Work out the finished part from the listing and answer in its coordinate system (mm). Face numbers are marked on the shaded views. A direction names the side the tool comes from. Round coordinates to 2 decimals unless told otherwise and drop trailing zeros. Loops run counter-clockwise (first coordinate to the right, second up) from the corner with the lowest first, then second, coordinate; pieces in that order, holes last. Notation, with made-up numbers: (-11.5, -35) -> (45.5, -35) arc R27 ccw to (45.5, -2) -> close; hole circle Ø10 at (11, 32.25). An arc over 180 degrees is marked (long way). Use one line per item in the form item = value.
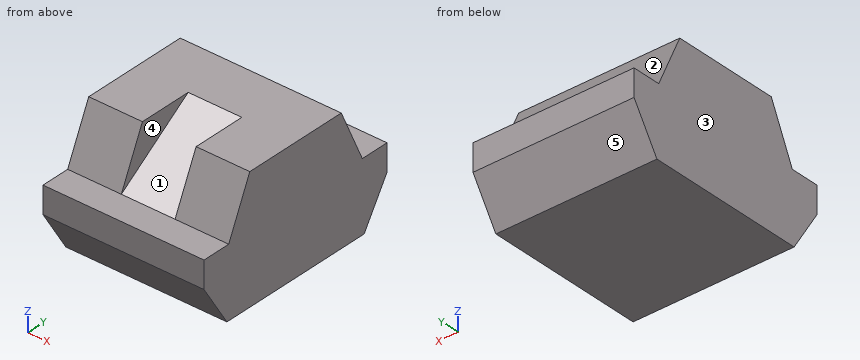
```python
from build123d import *

# Parameters (mm, degrees)
F1_DEPTH      = 76.2
F4_DEPTH      = 12.7
F4_DEPTH_BACK = 12.7


with BuildPart() as f1:
    # F0 (on Right) → F1 (new body)
    with BuildSketch(Plane.YZ):
        Polygon((-38.1, 0), (0, 0), (0, 58.3063843763), (-25.4, 58.3063843763), (-37.1005810608, 32.9063843763), (-50.8005463281, 32.9057950318), (-50.8, 20.2057950318), align=None)
        Polygon((0, 58.3063843763), (0, 0), (38.1, 0), (50.8, 20.2057950318), (50.8005463281, 32.9057950318), (37.1005810608, 32.9063843763), (25.4, 58.3063843763), align=None)
    extrude(amount=F1_DEPTH)

    # F3 (on mid) → F4 (cut, two sides)
    with BuildSketch(Plane.YZ.offset(38.1)) as f4_sk:
        Polygon((0, 58.3063843763), (-25.4, 58.3063843763), (-37.1005810608, 32.9063843763), align=None)
    extrude(amount=-F4_DEPTH, mode=Mode.SUBTRACT)
    extrude(f4_sk.sketch, amount=F4_DEPTH_BACK, mode=Mode.SUBTRACT)


solid = f1.part
```
(1) Consider L1, parallel to X at y = -13, z = 52.5; L2, parallel to Z at x = 64, y = -38; L3, parallel to Z at x = 51, y = 27.5. Determine where each line is inside the solid, lowest interval first.
Completed:
L1 = 0 to 25.4, 50.8 to 76.2
L2 = 0 to 32.91
L3 = 0 to 53.75
(2) Find section A-A, the plane x = 67.5. Write down the section's boundary in (y, z).
Completed:
outline = (-50.8, 20.21) -> (-38.1, 0) -> (38.1, 0) -> (50.8, 20.21) -> (50.8, 32.91) -> (37.1, 32.91) -> (25.4, 58.31) -> (-25.4, 58.31) -> (-37.1, 32.91) -> (-50.8, 32.91) -> close
(3) For the marked faces 4 and 5, determine the directions among +Z, -Z, +X, -X, +Y, -Y from which every point of the face is accessible in a straight line to the end or side of a thin tool.
Completed:
face_4 = +Z, -Y
face_5 = -Z, +X, -X, +Y
(4) For a pull along X with two mould halves and no side action, classify the marked faces 1, 2 and 3 as +X half, -X half, draft (parallel to the pull), parting line (faces both ways), or undercut.
Completed:
face_1 = undercut
face_2 = draft
face_3 = -X half
(5) Find section C-C, the plane z = 51. Write down the section's boundary in (x, y).
Completed:
outline = (0, -28.77) -> (25.4, -28.77) -> (25.4, -10.67) -> (50.8, -10.67) -> (50.8, -28.77) -> (76.2, -28.77) -> (76.2, 28.77) -> (0, 28.77) -> close
(6) Find section D-D, the plane x = 30.5. Write down the section's boundary in (y, z), then the cut area to 3 significant figures.
Completed:
outline = (-50.8, 20.21) -> (-38.1, 0) -> (38.1, 0) -> (50.8, 20.21) -> (50.8, 32.91) -> (37.1, 32.91) -> (25.4, 58.31) -> (0, 58.31) -> (-37.1, 32.91) -> (-50.8, 32.91) -> close
area = 4,350 mm2
(7) Given P1, Ø4, axis at x = 55.5, y = -45.5, coming from the +Z side; P2, Ø1, axis at x = 52.5, y = -30.5, coming from the +Z side; P3, Ø15, axis at x = 31.5, y = 41, coming from the +Z side, each flat-ended and moving along its own axis, determine where each tip first touches the part or whether it passes through.
Completed:
P1 = 32.91
P2 = 48.32
P3 = 40.72
(8) Find section B-B, the plane y = -16.5. Write down the section's boundary in (x, z).
Completed:
outline = (0, 0) -> (76.2, 0) -> (76.2, 58.31) -> (50.8, 58.31) -> (50.8, 47.01) -> (25.4, 47.01) -> (25.4, 58.31) -> (0, 58.31) -> close
